Can you work these out from the model? Positions are in its coordinate system, mm. Round coordinates to 2 decimals unless told otherwise and drop trailing zeros. Loops run counter-clockwise (first coordinate to the right, second up) from the corner with the lowest first, then second, coordinate; pieces in that order, holes last. Notation, with made-up numbers: M -33,-34.75 L -14,-34.75 A18 cw -14,-18.75 Z; hole C 40,29 d8. An arc over 180 degrees is marked long. Return JSON: item names as keys, results as strings.
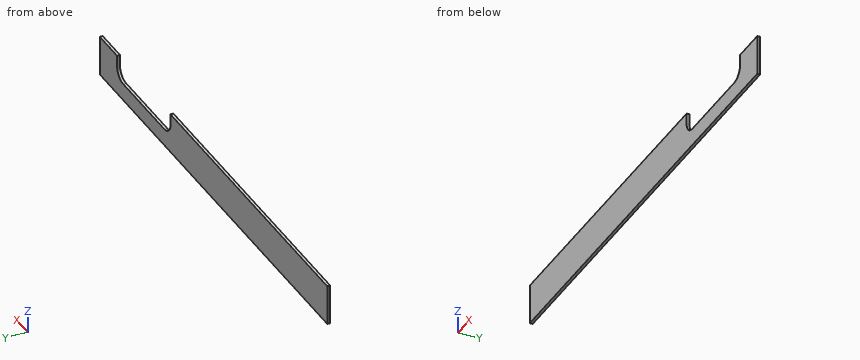
```python
from build123d import *

# Parameters (mm, degrees)
F0_W     = 2438.4
F0_H     = 88.9
F1_DEPTH = 6.35
F3_DEPTH = 6.351
F4_R     = 25.4
F5_W     = 1462.224513
F5_H     = 88.9
F6_DEPTH = 6.351


with BuildPart() as f1:
    # F0 (on Front) → F1 (new body)
    with BuildSketch(Plane.XZ):
        with Locations((1219.2, 44.45)):
            Rectangle(F0_W, F0_H)
    extrude(amount=F1_DEPTH)

    # F2 (on face) → F3 (cut, through all)
    with BuildSketch(Plane.XZ.offset(6.35)):
        Polygon((901.7, 88.9), (673.1, 88.9), (673.1, 38.1), (787.4, 38.1), (901.7, 38.1), align=None)
    extrude(amount=-F3_DEPTH, mode=Mode.SUBTRACT)

    # F4
    f4_edges = [f1.edges().sort_by_distance(p)[0] for p in [
        (673.1, -3.175, 38.1),
        (901.7, -3.175, 38.1),
    ]]
    fillet(f4_edges, radius=F4_R)

    # F5 (on face) → F6 (cut, through all)
    with BuildSketch(Plane.XZ.offset(6.35)):
        with Locations((1707.287744, 44.45)):
            Rectangle(F5_W, F5_H)
    extrude(amount=-F6_DEPTH, mode=Mode.SUBTRACT)


solid = f1.part
```
Q1. I'm going to push flat-ended pins straight in: pin 1 Ø1 at (x, y) = (335, -1) entering from -Z; pin 2 Ø1 at (x, y) = (720, -3.5) entering from +Z. Where does each tip first touch, or does it pass through?
Results:
{"pin 1": "stops at z = 0", "pin 2": "stops at z = 38.1"}
Q2. Suppose I cut it at C-C, the plane x = 723. Please give me the cut outline in (y, z), plus the area to 3 significant figures.
Results:
{"outline": "M -6.35,0 L 0,0 L 0,38.1 L -6.35,38.1 Z", "area": "242 mm2"}
Q3. If I drill on line 1 along X through (y, z) = (-5.5, 67.5); line 2 along Z through (x, y) = (815, -3.25), over which ranges is the centre line in solid material (lowest first)?
Results:
{"line 1": "x = 0 to 673.1, 901.7 to 976.18", "line 2": "z = 0 to 38.1"}
Q4. Suppose I cut it at A-A, the plane y = -2.5. Please give me the cut outline in (x, z), plus the area to 3 significant figures.
Results:
{"outline": "M 0,0 L 976.18,0 L 976.18,88.9 L 901.7,88.9 L 901.7,63.5 A25.4 cw 876.3,38.1 L 698.5,38.1 A25.4 cw 673.1,63.5 L 673.1,88.9 L 0,88.9 Z", "area": "75,400 mm2"}
Q5. Suppose I cut it at B-B, the plane z = 48. Please give me the cut outline in (x, y), plus the area to 3 significant figures.
Results:
{"outline": "M 0,-6.35 L 678.38,-6.35 L 678.38,0 L 0,0 Z; M 896.42,-6.35 L 976.18,-6.35 L 976.18,0 L 896.42,0 Z", "area": "4,810 mm2"}
